Check sheet for the modelled part. Datum: model origin and axes. Units: mm. A direction names the side the tool comes from. Give positions to 0.01 mm unless a question says otherwise; leave off trailing zeros. Write each loop counter-clockwise with the first axis right and the second up, starting at its lowest first coordinate (ties: lowest second). Pieces come first, ordered by that corner, then holes. Notation, with made-up numbers: M 26,30.5 L 53,30.5 A16 cw 53,53.5 Z; hole C -13.5,-0.5 d6. An arc over 180 degrees is marked long. Write item = value, one per line. Start each with the question number.
1) Draft check along X on faces 1 (the face through (20.09, 11.29, 2.46)), 2 (the face through (0, -4, 0)), 3 (the face through (0.13, 27.67, 2.46)). Enter one of: pulls with the +X half, pulls with the -X half, needs draft (parallel to the pull), parting line crosses it, or undercut.
2) Sectioned sample at D-D, the plane x = -1. Record the cut outline in (y, z), then the cut area to 3 significant figures.
3) Sectioned sample at B-B, the plane z = 1.6. Record the cut outline in (x, y).
4) Sectioned sample at C-C, the plane y = 3. Record the cut outline in (x, z).
5) Scan lines: L1, parallel to Z at x = -19.5, y = 3; L2, parallel to X at y = 13.5, z = 3.15; L3, parallel to Y at x = -13, z = 2.3. Record each from-to range of solid material in increasing order.
6) Set-up check for faces 4 (the face through (-19.8, 11.8, 2.5)), 5 (the face through (-21.43, -12.22, 3.99)): record each of +Z, -Z, +X, -X, +Y, -Y from which the full face is reachable in a straight line by a thin tool's end or side.
7) Gauge pin test, flat ends, axial feed: pin 1 (6 mm diameter, centred on x = 1, y = -6, fed in from +Z); pin 2 (2 mm diameter, centred on y = 4.5, z = 0.5, fed in from -X); pin 3 (3 mm diameter, centred on y = -1.5, z = 3.5, fed in from +X). Record the tip position at first contact, or that the pin passes through.
8) Sectioned sample at A-A, the plane x = -32. Record the cut outline in (y, z), then the cut area to 3 significant figures.
from build123d import *

# Parameters (mm, degrees)
F2_DEPTH    = 5
F3_D        = 2.2606
F4_T        = 3
F4_T3_DEPTH = 11


# Not quite as in the source:
# - a shell that OpenCascade refuses in one call is made with other operations: the cavity is built on its own and cut out


with BuildPart() as f2:
    # F1 (on Top) → F2 (new body)
    with BuildSketch(Plane.XY):
        with BuildLine():
            ThreePointArc((9, 30.0222139979), (0, 27.6692232402), (-9, 30.0222139979))
            ThreePointArc((-9, 30.0222139979), (-12, 33.0222139979), (-15, 30.0222139979))
            ThreePointArc((-15, 30.0222139979), (-19.95706006, 11.5222139979), (-33.5, -2.0207259422))
            ThreePointArc((-33.5, -2.0207259422), (-34.5980762114, -6.1188021535), (-30.5, -7.2168783649))
            ThreePointArc((-30.5, -7.2168783649), (-23.962250229, -13.8346116201), (-21.5, -22.805335633))
            ThreePointArc((-21.5, -22.805335633), (-22.5980762114, -26.9034118443), (-18.5, -28.0014880557))
            ThreePointArc((-18.5, -28.0014880557), (0, -23.0444279957), (18.5, -28.0014880557))
            ThreePointArc((18.5, -28.0014880557), (22.5980762114, -26.9034118443), (21.5, -22.805335633))
            ThreePointArc((21.5, -22.805335633), (23.962250229, -13.8346116201), (30.5, -7.2168783649))
            ThreePointArc((30.5, -7.2168783649), (34.5980762114, -6.1188021535), (33.5, -2.0207259422))
            ThreePointArc((33.5, -2.0207259422), (19.95706006, 11.5222139979), (15, 30.0222139979))
            ThreePointArc((15, 30.0222139979), (12, 33.0222139979), (9, 30.0222139979))
        make_face()
    extrude(amount=F2_DEPTH)

    # F3 (through all)
    with Locations(Plane(origin=(0, 0, 0), x_dir=(1, 0, 0), z_dir=(0, 0, -1))):
        with Locations((-12, -30.0222139979), (12, -30.0222139979), (32, 4.6188021535), (20, 25.4034118443), (-20, 25.4034118443), (-32, 4.6188021535)):
            Hole(F3_D / 2)

    # F4: shell of thickness 3, made by hand


with BuildPart() as f4_core1:
    # F4_t2: copy of F2
    add(f2.part)

    # the walls: a layer under each face that stays
    f4_faces = [f4_core1.faces().sort_by_distance(p)[0] for p in [
        (0, -23.0444279957, 2.5),
        (0, 2.3094010768, 0),
        (-23.962250229, -13.8346116201, 2.5),
        (23.962250229, -13.8346116201, 2.5),
        (-19.95706006, 11.5222139979, 2.5),
        (19.95706006, 11.5222139979, 2.5),
        (0, 27.6692232402, 2.5),
        (-21.1303, -25.4034118443, 2.5),
        (-33.1303, -4.6188021535, 2.5),
        (18.8697, -25.4034118443, 2.5),
        (30.8697, -4.6188021535, 2.5),
        (-13.1303, 30.0222139979, 2.5),
        (10.8697, 30.0222139979, 2.5),
    ]]
    thicken(f4_faces, amount=-F4_T, mode=Mode.SUBTRACT)

    # F4_s4 → F4_t3 (cut)
    with BuildSketch(Plane.XY.offset(-3)):
        Polygon((-21.5449977822, -22.7797196489), (-20, -25.4034118443), (-18.4788645602, -24.5251838887), (-18.5002217799, -22.7688578263), align=None)
        Polygon((21.5449977822, -22.7797196489), (20, -25.4034118443), (18.4788645602, -24.5251838887), (18.5002217799, -22.7688578263), align=None)
        Polygon((-30.5003147982, -7.2686555794), (-28.9685201827, -4.6372331239), (-30.4788645602, -3.7405741979), (-32, -4.6188021535), align=None)
        Polygon((30.5003147982, -7.2686555794), (28.9685201827, -4.6372331239), (30.4788645602, -3.7405741979), (32, -4.6188021535), align=None)
        Polygon((-8.955317016, 30.0483752283), (-12, 30.0222139979), (-12, 28.2657580866), (-10.4682984028, 27.4060909502), align=None)
        Polygon((8.955317016, 30.0483752283), (12, 30.0222139979), (12, 28.2657580866), (10.4682984028, 27.4060909502), align=None)
    extrude(amount=F4_T3_DEPTH, mode=Mode.SUBTRACT)


with BuildPart() as f2_1:
    add(f2.part)

    # what is left inside the walls is the cavity
    f4_cavity = [f4_core1.part.solids().sort_by_distance(p)[0] for p in [
        (0, -6.739348, 4.97),
    ]]
    add(f4_cavity, mode=Mode.SUBTRACT)


solid = f2_1.part
Data:
q1.face_1 = pulls with the +X half
q1.face_2 = needs draft
q1.face_3 = undercut
q2.outline = M -23.06,0 L 27.7,0 L 27.7,5 L 24.69,5 L 24.69,3 L -20.06,3 L -20.06,5 L -23.06,5 Z
q2.area = 164 mm2
q3.outline = M -33.5,-2.02 A3 ccw -30.5,-7.22 A18.39 cw -21.5,-22.81 A3 ccw -18.5,-28 A37 cw 18.5,-28 A3 ccw 21.5,-22.81 A18.39 cw 30.5,-7.22 A3 ccw 33.5,-2.02 A37 cw 15,30.02 A3 ccw 9,30.02 A18.39 cw -9,30.02 A3 ccw -15,30.02 A37 cw Z; hole C -32,-4.62 d2.26; hole C -20,-25.4 d2.26; hole C -12,30.02 d2.26; hole C 12,30.02 d2.26; hole C 20,-25.4 d2.26; hole C 32,-4.62 d2.26
q4.outline = M -26.73,0 L 26.73,0 L 26.73,5 L 22.51,5 L 22.51,3 L -22.51,3 L -22.51,5 L -26.73,5 Z
q5.L1 = 0 to 3
q5.L2 = -18.89 to -15.57, 15.57 to 18.89
q5.L3 = -25.4 to 29.5, 30.55 to 32.85
q6.face_4 = +Z, -Z, -X, +Y
q6.face_5 = +Z
q7.pin_1 = 3
q7.pin_2 = -26.2
q7.pin_3 = 34.53
q8.outline = M -7.62,0 L -5.75,0 L -5.75,5 L -7.62,5 Z; M -3.49,0 L -1.11,0 L -1.11,5 L -3.49,5 Z
q8.area = 21.3 mm2
